For this review, use the dimensioned drawing (mm, ordinates from the lowest corner) and the shaded views. Round coordinates to 2 decimals unless told otherwise and drop trailing zeros. Order: outer loops, then holes, each group sorted by start corner. A loop starts at its lowest first (then second) coordinate and runs counter-clockwise, first axis right, second up. Notation, with made-up numbers: M 78.5,-33 L 91.5,-33 A26 cw 91.5,-14 Z; hole C 85.5,3.5 d1. An arc over 180 degrees is marked long. Put each result on its own line as item: value.
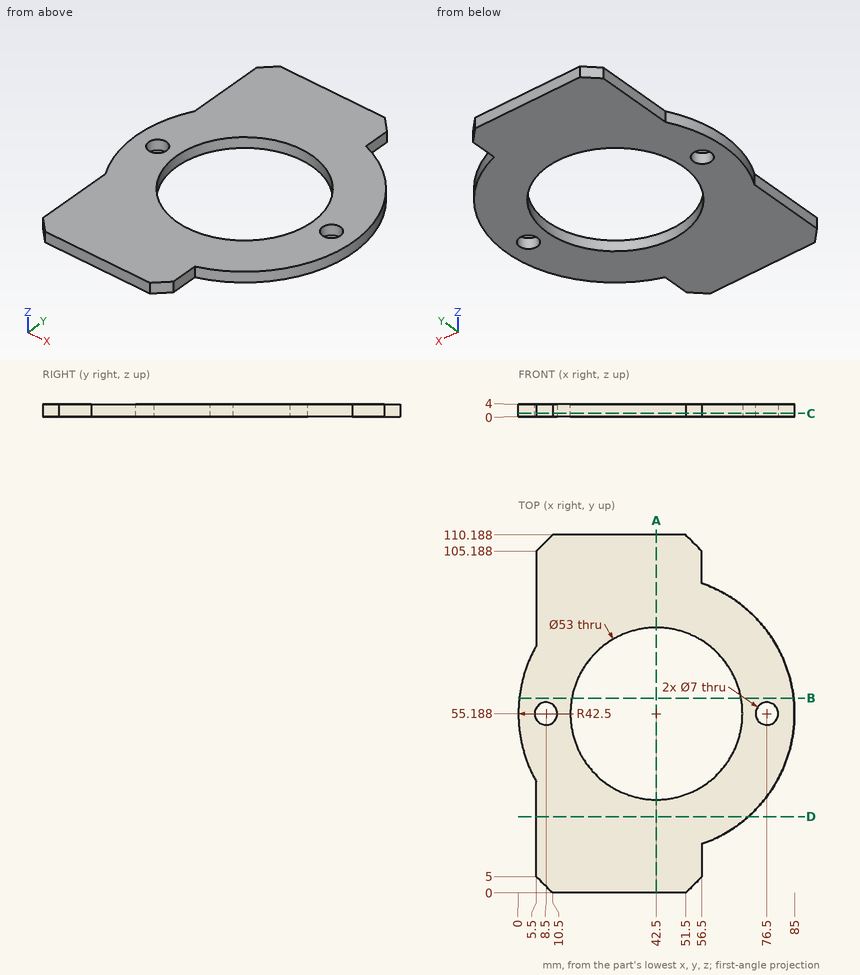
(1) Add section D-D on y = 23.5. Give the boundary of the cut face in (x, z), then the cut area to 3 significant figures.
A:
outline: M 5.5,0 L 70.82,0 L 70.82,4 L 5.5,4 Z
area: 261 mm2
(2) Add section A-A on x = 42.5. Give the boundary of the cut face in (y, z), then the cut area to 3 significant figures.
A:
outline: M 0,0 L 28.69,0 L 28.69,4 L 0,4 Z; M 81.69,0 L 110.19,0 L 110.19,4 L 81.69,4 Z
area: 229 mm2
(3) Add section B-B on y = 60. Give the boundary of the cut face in (x, z).
A:
outline: M 0.27,0 L 16.44,0 L 16.44,4 L 0.27,4 Z; M 68.56,0 L 84.73,0 L 84.73,4 L 68.56,4 Z
(4) To check wall thickness, follow L1, parallel to X at y = 55.5, z = 0.45; L2, parallel to Y at x = 42.5, z = 1.1; L3, parallel to X at y = 56.5, z = 1.35 (1 decimal). State the ranges of each line that lie inside material, in increasing order.
A:
L1: x = 0 to 5.01, 11.99 to 16, 69 to 73.01, 79.99 to 85
L2: y = 0 to 28.69, 81.69 to 110.19
L3: x = 0 to 5.3, 11.7 to 16, 69 to 73.3, 79.7 to 85
(5) Add section C-C on z = 1.1. Give the boundary of the cut face in (x, y).
A:
outline: M 5.5,5 L 10.5,0 L 51.5,0 L 56.5,5 L 56.5,15.06 A42.5 ccw 56.5,95.32 L 56.5,105.19 L 51.5,110.19 L 10.5,110.19 L 5.5,105.19 L 5.5,76.1 A42.5 ccw 5.5,34.28 Z; hole C 8.5,55.19 d7; hole C 42.5,55.19 d53; hole C 76.5,55.19 d7
(6) Insertion check: pin 1 Ø1.2 at (y, z) = (10.5, 1.5) entering from +X; pin 2 Ø1.5 at (y, z) = (81.5, 2) entering from -X. Each pin has a flat end and moves straight along its axis. Give the tip position at first contact, or say it passes through.
A:
pin 1: stops at x = 56.5
pin 2: stops at x = 5.5
